Autodesk Inventor part; units mm, degrees
ref_plane "YZ Plane" through (0, 0, 0) normal (1, 0, 0) x (0, 1, 0)
ref_plane "XZ Plane" through (0, 0, 0) normal (0, 1, 0) x (-1, 0, 0)
ref_plane "XY Plane" through (0, 0, 0) normal (0, 0, 1) x (1, 0, 0)
sketch "Sketch2" plane through (0, 0, 0) normal (0, 1, 0) x (-1, 0, 0)
  line L0 (-46, -50) -> (46, -50)
  line L1 (50, -46) -> (50, 46)
  line L2 (46, 50) -> (-46, 50)
  line L3 (-50, 46) -> (-50, -46)
  line L4 (-50, -50) -> (50, 50) construction
  line L5 (50, -50) -> (-50, 50) construction
  arc A0 (50, 46) -> (46, 50) centre (46, 46) ccw
  arc A1 (-46, 50) -> (-50, 46) centre (-46, 46) ccw
  arc A2 (-50, -46) -> (-46, -50) centre (-46, -46) ccw
  arc A3 (46, -50) -> (50, -46) centre (46, -46) ccw
  point P0 (0, 0)
  dimension "d0" = 100
  dimension "d1" = 100
  dimension "d4" = 4
  dimension "d5" = 4
extrude "Extrusion1" add sketch "Sketch2" along normal blind 5
sketch "Sketch3" plane through (0, 0, 0) normal (0, -1, 0) x (1, 0, 0)
  arc A0 (-50, -46) -> (-46, -50) centre (-46, -46) ccw construction
  line L0 (46, -50) -> (-46, -50) construction
  arc A1 (46, -50) -> (50, -46) centre (46, -46) ccw construction
  line L1 (50, 46) -> (50, -46) construction
  arc A2 (50, 46) -> (46, 50) centre (46, 46) ccw construction
  line L2 (-46, 50) -> (46, 50) construction
  arc A3 (-46, 50) -> (-50, 46) centre (-46, 46) ccw construction
  line L3 (-50, -46) -> (-50, 46) construction
  point P0 (0, 0)
  point P1 (-45, 45)
  point P2 (45, 45)
  point P3 (-45, -45)
  point P4 (45, -45)
  dimension "d13" = 5
  dimension "d14" = 5
  dimension "d17" = 90
  dimension "d20" = 90
hole "Hole1" at (-45, 0, 45) at (45, 0, 45) at (45, 0, -45) at (-45, 0, -45) direction (0, 1, 0) diameter 5 depth 14.2 tip angle 118
sketch "Sketch4" plane through (0, 5, 0) normal (0, 1, 0) x (1, 0, 0)
  circle A0 centre (45, 45) radius 2.5 construction
  circle A1 centre (-45, -45) radius 2.5 construction
  circle A2 centre (45, -45) radius 2.5 construction
  circle A3 centre (-45, 45) radius 2.5 construction
  arc A4 (-46, 50) -> (-50, 46) centre (-46, 46) ccw construction
  line L0 (-50, 46) -> (-50, -46) construction
  arc A5 (-50, -46) -> (-46, -50) centre (-46, -46) ccw construction
  line L1 (-46, -50) -> (46, -50) construction
  arc A6 (46, -50) -> (50, -46) centre (46, -46) ccw construction
  line L2 (50, -46) -> (50, 46) construction
  arc A7 (50, 46) -> (46, 50) centre (46, 46) ccw construction
  line L3 (46, 50) -> (-46, 50) construction
  arc A8 (44.6333, -39.5122) -> (39.5122, -44.6333) centre (45, -45) ccw
  arc A9 (45.9545, -41.6327) -> (41.6327, -45.9545) centre (45, -45) ccw
  line L4 (39.7085, -48.5) -> (-39.7085, -48.5)
  line L5 (48.5, -39.7085) -> (48.5, 39.7085)
  line L6 (46.5, -37.5167) -> (46.5, 37.5167)
  line L7 (0, -72.209) -> (0, 64.6676) construction
  line L8 (107.9328, 0) -> (-102.5907, 0) construction
  line L9 (37.5167, -46.5) -> (-37.5167, -46.5)
  arc A10 (-39.5122, -44.6333) -> (-44.6333, -39.5122) centre (-45, -45) ccw
  arc A11 (-41.6327, -45.9545) -> (-45.9545, -41.6327) centre (-45, -45) ccw
  line L10 (-48.5, -39.7085) -> (-48.5, 39.7085)
  line L11 (-46.5, 37.5167) -> (-46.5, -37.5167)
  arc A12 (41.6327, 45.9545) -> (45.9545, 41.6327) centre (45, 45) ccw
  arc A13 (39.5122, 44.6333) -> (44.6333, 39.5122) centre (45, 45) ccw
  line L12 (39.7085, 48.5) -> (-39.7085, 48.5)
  line L13 (37.5167, 46.5) -> (-37.5167, 46.5)
  line L14 (46, 50) -> (-46, 50) construction
  arc A14 (-44.6333, 39.5122) -> (-39.5122, 44.6333) centre (-45, 45) ccw
  arc A15 (-45.9545, 41.6327) -> (-41.6327, 45.9545) centre (-45, 45) ccw
  arc A16 (39.7085, -48.5) -> (41.6327, -45.9545) centre (39.7085, -46.5) ccw
  arc A17 (37.5167, -46.5) -> (39.5122, -44.6333) centre (37.5167, -44.5) ccw
  arc A18 (45.9545, -41.6327) -> (48.5, -39.7085) centre (46.5, -39.7085) ccw
  arc A19 (44.6333, -39.5122) -> (46.5, -37.5167) centre (44.5, -37.5167) ccw
  arc A20 (-41.6327, -45.9545) -> (-39.7085, -48.5) centre (-39.7085, -46.5) ccw
  arc A21 (-39.5122, -44.6333) -> (-37.5167, -46.5) centre (-37.5167, -44.5) ccw
  arc A22 (-48.5, -39.7085) -> (-45.9545, -41.6327) centre (-46.5, -39.7085) ccw
  arc A23 (-46.5, -37.5167) -> (-44.6333, -39.5122) centre (-44.5, -37.5167) ccw
  arc A24 (-44.6333, 39.5122) -> (-46.5, 37.5167) centre (-44.5, 37.5167) ccw
  arc A25 (-45.9545, 41.6327) -> (-48.5, 39.7085) centre (-46.5, 39.7085) ccw
  arc A26 (-39.7085, 48.5) -> (-41.6327, 45.9545) centre (-39.7085, 46.5) ccw
  arc A27 (-37.5167, 46.5) -> (-39.5122, 44.6333) centre (-37.5167, 44.5) ccw
  arc A28 (41.6327, 45.9545) -> (39.7085, 48.5) centre (39.7085, 46.5) ccw
  arc A29 (39.5122, 44.6333) -> (37.5167, 46.5) centre (37.5167, 44.5) ccw
  arc A30 (48.5, 39.7085) -> (45.9545, 41.6327) centre (46.5, 39.7085) ccw
  arc A31 (46.5, 37.5167) -> (44.6333, 39.5122) centre (44.5, 37.5167) ccw
  point P0 (0, 0)
  point P1 (45, -48.5)
  point P2 (39.7085, -46.5)
  point P3 (48.5, -45)
  point P4 (48.5, 45)
  point P5 (46.5, -39.7085)
  point P6 (46.5, 39.7085)
  point P7 (-45, -48.5)
  point P8 (-48.5, -45)
  point P9 (-46.5, 39.7085)
  point P10 (-46.5, -39.7085)
  point P11 (45, 48.5)
  point P12 (-45, 48.5)
  point P13 (39.7085, 46.5)
  point P14 (-39.7085, 46.5)
  point P15 (-48.5, 45)
  dimension "d23" = 5.5
  dimension "d24" = 3.5
  dimension "d25" = 1.5
  dimension "d27" = 1.5
  dimension "d28" = 2
  dimension "d31" = 5.5
  dimension "d32" = 3.5
  dimension "d33" = 2
  dimension "d34" = 1.5
  dimension "d35" = 2
  dimension "d36" = 5.5
  dimension "d37" = 3.5
  dimension "d38" = 1.5
  dimension "d39" = 2
  dimension "d41" = 5.5
  dimension "d42" = 3.5
  dimension "d43" = 2
  dimension "d44" = 2
  dimension "d45" = 2
extrude "Extrusion2" cut sketch "Sketch4" against normal blind 2
sketch "Sketch5" plane through (0, 0, 0) normal (0, -1, 0) x (1, 0, 0)
  circle A0 centre (45, -45) radius 2.5 construction
  circle A1 centre (-45, 45) radius 2.5 construction
  circle A2 centre (45, 45) radius 2.5 construction
  circle A3 centre (-45, -45) radius 2.5 construction
  arc A4 (-50, -46) -> (-46, -50) centre (-46, -46) ccw construction
  line L0 (46, -50) -> (-46, -50) construction
  arc A5 (46, -50) -> (50, -46) centre (46, -46) ccw construction
  line L1 (50, 46) -> (50, -46) construction
  arc A6 (50, 46) -> (46, 50) centre (46, 46) ccw construction
  line L2 (-46, 50) -> (46, 50) construction
  arc A7 (-46, 50) -> (-50, 46) centre (-46, 46) ccw construction
  line L3 (-50, -46) -> (-50, 46) construction
  arc A8 (-1.7321, 2.75) -> (1.7321, 2.75) centre (0, 0) ccw
  line L4 (-1.7321, 2.75) -> (1.7321, 2.75)
  dimension "d48" = 50
  dimension "d49" = 50
  dimension "d50" = 6.5
  dimension "d51" = 6
extrude "Extrusion3" cut sketch "Sketch5" against normal through all
properties part number "P035_FondBoitierv3"
Could you check a few things on this model? Use its own coordinates, in mm. A direction names the side the tool comes from. Give positions to 0.01 mm unless a question says otherwise; leave off trailing zeros. Loops run counter-clockwise (first coordinate to the right, second up) from the corner with the lowest first, then second, coordinate; pieces in that order, holes last. Notation, with made-up numbers: (-30, -10.5) - (14, -10.5) arc R29 ccw to (14, 10.5) - close; hole circle Ø8 at (56.25, -2). An arc over 180 degrees is marked (long way). Use one line per item in the form item = value.
1. I want a section at D-D (z = -32). Please give me the cut outline in (x, y), and give its area (3 significant figures).
Response values:
outline = (-50, 0) - (50, 0) - (50, 5) - (48.5, 5) - (48.5, 3) - (46.5, 3) - (46.5, 5) - (-46.5, 5) - (-46.5, 3) - (-48.5, 3) - (-48.5, 5) - (-50, 5) - close
area = 492 mm²
2. I'm going to push a flat-ended pin straight in: pin 1 Ø4.5 at (x, z) = (-45, -45) entering from -Y. Where does the tip first touch, or does it pass through?
Response values:
pin_1 = through
3. Thinking about a two-plate mould opening in X: for faces 4 (the face through (-41.07, 4.01, 41.15)), 5 (the face through (-48.797, 2.465, 48.859)), 6 (the face through (1, 2, -50)), 7 (the face through (48.859, 2.465, 48.797)), which applies, released by +X, released by -X, zero draft, split by the parting line, or undercut?
Response values:
face_4 = undercut
face_5 = released by -X
face_6 = zero draft
face_7 = released by +X
4. On a 3-axis mill with a long thin cutter (end or side, diameter ignored), from which of +Z, -Z, +X, -X, +Y, -Y can I reach the whole of each face in a straight line? I mean faces 1 (the face through (-18, 3, -47)), 2 (the face through (0, 2, 2.75)), 3 (the face through (1, 5, -10)). Say none if no direction works.
Response values:
face_1 = +Y
face_2 = +Y, -Y
face_3 = +Z, -Z, +X, -X, +Y
5. I need wall thicknesses on probe 1 along Z at (x, y) = (-8.5, 3.1); probe 2 along Z at (x, y) = (45, 1). Which ranges of each line are inside material? Lowest first, please.
Response values:
probe_1 = -50 to -48.5, -46.5 to 46.5, 48.5 to 50
probe_2 = -50 to -47.5, -42.5 to 42.5, 47.5 to 50
6. I want a section at B-B (z = 0). Please give me the cut outline in (x, y), and give its area (4 significant figures).
Response values:
outline = (-50, 0) - (-3.25, 0) - (-3.25, 5) - (-46.5, 5) - (-46.5, 3) - (-48.5, 3) - (-48.5, 5) - (-50, 5) - close; (3.25, 0) - (50, 0) - (50, 5) - (48.5, 5) - (48.5, 3) - (46.5, 3) - (46.5, 5) - (3.25, 5) - close
area = 459.5 mm²
7. I want a section at A-A (x = 0). Please give me the cut outline in (y, z), and give its area (3 significant figures).
Response values:
outline = (0, -50) - (5, -50) - (5, -48.5) - (3, -48.5) - (3, -46.5) - (5, -46.5) - (5, -3.25) - (0, -3.25) - close; (0, 2.75) - (5, 2.75) - (5, 46.5) - (3, 46.5) - (3, 48.5) - (5, 48.5) - (5, 50) - (0, 50) - close
area = 462 mm²
8. I want a section at C-C (x = 31). Please give me the cut outline in (y, z).
Response values:
outline = (0, -50) - (5, -50) - (5, -48.5) - (3, -48.5) - (3, -46.5) - (5, -46.5) - (5, 46.5) - (3, 46.5) - (3, 48.5) - (5, 48.5) - (5, 50) - (0, 50) - close
